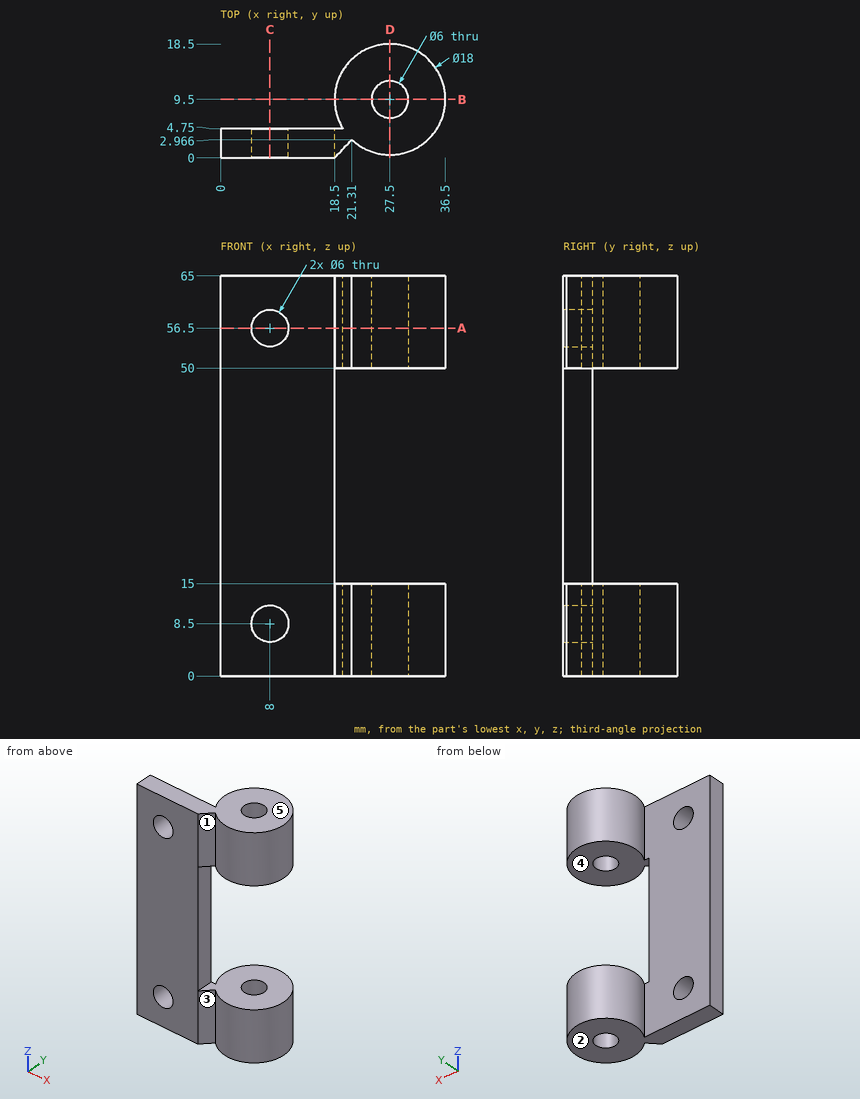
The figure shows three views and two pictorial views of one solid part (mm, origin at its lowest corner). Answer the questions. A direction names the side the tool comes from. Give positions to 0.01 mm unless a question says otherwise; leave off trailing zeros. Order: outer loops, then holes, each group sorted by start corner. A loop starts at its lowest first (then second) coordinate and runs counter-clockwise, first axis right, second up. Notation, with made-up numbers: (12.5, 33) -> (58.5, 33) arc R20 ccw to (58.5, 69) -> close; hole circle Ø6 at (84.25, 36). An arc over 180 degrees is marked (long way). Answer as a JSON object with one key per item and string values. Group by question number.
Item 1: Consider L1, parallel to Z at x = 23, y = 4.25; L2, parallel to Y at x = 27.5, z = 58; L3, parallel to X at y = 2, z = 7 (1 decimal). Determine where each line is inside the solid, lowest interval first. Write a range as from..to.
Item 2: The part is cut by section B-B on y = 9.5. Write down the section's boundary in (x, z), and give its area (3 significant figures).
Item 3: The part is cut by section A-A on z = 56.5. Give the number of separate pieces and of enclosed holes in the cut face, and give its area (3 significant figures).
Item 4: The part is cut by section D-D on x = 27.5. Write down the section's boundary in (y, z), and give its area (3 significant figures).
Item 5: A tool of negligible diameter and unlimited length cuts with its end or side. For the marked faces 4 and 5, from which of +Z, -Z, +X, -X, +Y, -Y can it reach the whole face along a straight path? Write none if from no direction.
Item 6: Determine the mould class of the marked faces 1, 2 and 3 for opening direction X: pulls with the +X half, pulls with the -X half, needs draft (parallel to the pull), parting line crosses it, or undercut.
Item 7: Flat-ended cylindrical pins translate along their axes: pin 1 (5 mm diameter, centred on y = 3, z = 27, fed in from +X); pin 2 (8 mm diameter, centred on x = 9.5, z = 20, fed in from +Y); pin 3 (1 mm diameter, centred on x = 19.5, z = 7.5, fed in from -Y). Find the tip coordinate at first contact, or state that the pin passes through.
Item 8: The part is cut by section C-C on x = 8. Write down the section's boundary in (y, z), and give its area (3 significant figures).
Result set:
{
 "1": {"L1": "0..15, 50..65", "L2": "0.5..6.5, 12.5..18.5", "L3": "0..5.4, 10.6..20.4, 22.5..32.5"},
 "2": {"outline": "(18.5, 0) -> (24.5, 0) -> (24.5, 15) -> (18.5, 15) -> close; (18.5, 50) -> (24.5, 50) -> (24.5, 65) -> (18.5, 65) -> close; (30.5, 0) -> (36.5, 0) -> (36.5, 15) -> (30.5, 15) -> close; (30.5, 50) -> (36.5, 50) -> (36.5, 65) -> (30.5, 65) -> close", "area": "360 mm²"},
 "3": {"separate pieces": "2", "enclosed holes": "1", "area": "293 mm²"},
 "4": {"outline": "(0.5, 0) -> (6.5, 0) -> (6.5, 15) -> (0.5, 15) -> close; (0.5, 50) -> (6.5, 50) -> (6.5, 65) -> (0.5, 65) -> close; (12.5, 0) -> (18.5, 0) -> (18.5, 15) -> (12.5, 15) -> close; (12.5, 50) -> (18.5, 50) -> (18.5, 65) -> (12.5, 65) -> close", "area": "360 mm²"},
 "5": {"face 4": "+X, +Y, -Y", "face 5": "+Z, +X, -X, +Y, -Y"},
 "6": {"face 1": "undercut", "face 2": "needs draft", "face 3": "undercut"},
 "7": {"pin 1": "x = 18.5", "pin 2": "y = 4.75", "pin 3": "y = 0.53"},
 "8": {"outline": "(0, 0) -> (4.75, 0) -> (4.75, 5.5) -> (0, 5.5) -> close; (0, 11.5) -> (4.75, 11.5) -> (4.75, 53.5) -> (0, 53.5) -> close; (0, 59.5) -> (4.75, 59.5) -> (4.75, 65) -> (0, 65) -> close", "area": "252 mm²"}
}
